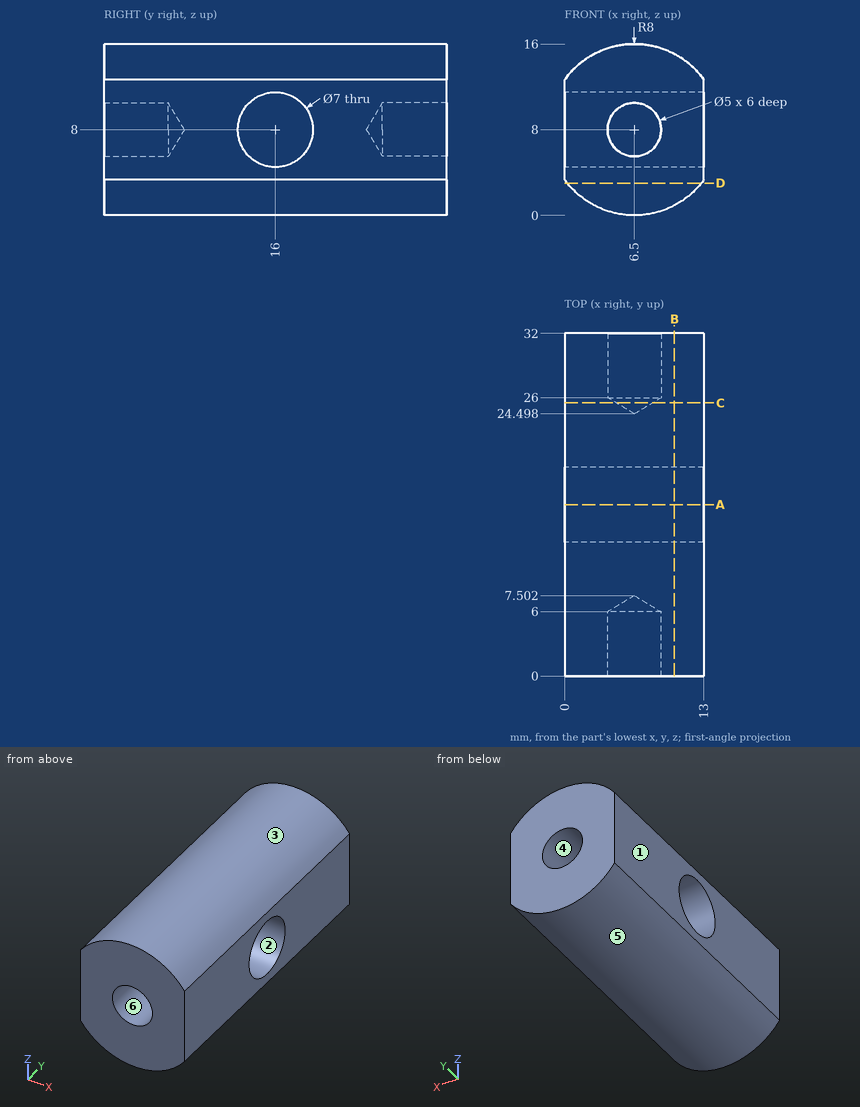
Source: three-view drawing plus pictorial views. Frame: mm from the lowest corner of the part. A direction names the side the tool comes from. Round coordinates to 2 decimals unless told otherwise and drop trailing zeros. Loops run counter-clockwise (first coordinate to the right, second up) from the corner with the lowest first, then second, coordinate; pieces in that order, holes last.
Q1. Section D-D, the plane z = 3. Return loops of the section in (x, y) (3 decimals), plus the area to 3 significant figures.
Q2. Ray query, line 1 (Z direction, x = 6.5, y = 29.3); line 2 (X direction, y = 4.45, z = 8); line 3 (Z direction, x = 1.75, y = 13.5). Return the intervals inside material, ascending.
Q3. Section B-B, the plane x = 10.25. Return loops of the section in (y, z).
Q4. First-contact query: P1, Ø2, axis at x = 11, y = 24.5, coming from the +Z side; P2, Ø1, axis at x = 7.5, y = 27.5, coming from the -Z side; P3, Ø3, axis at x = 6.5, z = 8, coming from the +Y side. Flat tips, straight axial feed; report the tip coordinate or a pass-through.
Q5. Section A-A, the plane y = 16. Return loops of the section in (x, z), plus the area to 3 significant figures.
Q6. Access query for the marked faces 4, 5 and 6. Directions: +Z, -Z, +X, -X, +Y, -Y. A direction counts if a zero-diameter tool reaches every point of the face in a straight line with its end or side. Return the directions, or none.
Q7. Mould query, pull axis Z, two halves, no side actions, for the marked faces 1, 2 and 3. Classes: pulls with the +Z half, pulls with the -Z half, needs draft (parallel to the pull), parting line crosses it, or undercut.
Q8. Section C-C, the plane y = 25.5. Return loops of the section in (x, z), plus the area to 3 significant figures.
Solutions:
1. outline: (0.255, 0) - (12.745, 0) - (12.745, 32) - (0.255, 32) - close
1. area: 400 mm2
2. line 1: z = 0 to 5.5, 10.5 to 16
2. line 2: x = 0 to 4, 9 to 13
2. line 3: z = 1.56 to 5.55, 10.45 to 14.44
3. outline: (0, 0.93) - (32, 0.93) - (32, 15.07) - (0, 15.07) - close; hole circle Ø7 at (16, 8)
4. P1: stops at z = 15.19
4. P2: stops at z = 0.02
4. P3: stops at y = 25.4
5. outline: (0, 3.34) arc R8 ccw to (13, 3.34) - (13, 4.5) - (0, 4.5) - close; (0, 11.5) - (13, 11.5) - (13, 12.66) arc R8 ccw to (0, 12.66) - close
5. area: 91.0 mm2
6. face 4: +Y
6. face 5: -Z, +Y, -Y
6. face 6: -Y
7. face 1: needs draft
7. face 2: undercut
7. face 3: pulls with the +Z half
8. outline: (0, 3.34) arc R8 ccw to (13, 3.34) - (13, 12.66) arc R8 ccw to (0, 12.66) - close; hole circle Ø3.34 at (6.5, 8)
8. area: 173 mm2
